from build123d import *

# Parameters (mm, degrees)
BOSS_EXTRUDE1_DEPTH = 15
CUT_EXTRUDE1_REACH  = 4
SKETCH3_R           = 1.5


with BuildPart() as part:
    # Sketch1 → Boss-Extrude1 (new body)
    with BuildSketch(Plane(origin=(0, 0, 0), x_dir=(0, 0, -1), z_dir=(1, 0, 0))):
        Polygon((0, 0), (16, 0), (16, -9), (26, -9), (26, -11), (14, -11), (14, -2), (0, -2), align=None)
    extrude(amount=-BOSS_EXTRUDE1_DEPTH)

    # Sketch3 → Cut-Extrude1 (cut, up to next)
    with BuildSketch(Plane(origin=(0, -9, 0), x_dir=(1, 0, 0), z_dir=(0, 1, 0)), mode=Mode.PRIVATE) as cut_extrude1_sk1:
        with Locations((-7.5, 21)):
            Circle(SKETCH3_R)
    cut_extrude1_tool1 = extrude(cut_extrude1_sk1.sketch, amount=-CUT_EXTRUDE1_REACH, mode=Mode.PRIVATE) & part.part
    add(cut_extrude1_tool1.solids().sort_by_distance((-7.5, -9, -21))[0], mode=Mode.SUBTRACT)


solid = part.part
The listing builds one solid part. Answer for the finished solid, in the listing's coordinates (mm). A direction names the side the tool comes from. Give positions to 0.01 mm unless a question says otherwise; leave off trailing zeros. Loops run counter-clockwise (first coordinate to the right, second up) from the corner with the lowest first, then second, coordinate; pieces in that order, holes last.
Item 1: A tool of negligible diameter and unlimited length cuts with its end or side. For faces 1 (the flat face through (-7, -2, -7)), 2 (the flat face through (-7, -4, -16)), 3 (the flat face through (-7, -10, -26)), from which of +Z, -Z, +X, -X, +Y, -Y can it reach the whole face along a straight path? Write none if from no direction.
Derived:
face 1: +Z, +X, -X, -Y
face 2: -Z, +X, -X, +Y
face 3: -Z, +X, -X, +Y, -Y
Item 2: Determine the mould class of faces 4 (the flat face through (-7, -1, 0)), 5 (the flat face through (-5.7, -9, -20.9)), 6 (the cylindrical face through (-8.61, -9.99, -22.01)) for opening direction Z: +Z half, -Z half, draft (parallel to the pull), parting line (faces both ways), or undercut.
Derived:
face 4: +Z half
face 5: draft
face 6: undercut
Item 3: A cutting plane is placed at A-A (x = -7.5). Give the vertices of the cut face in (y, z).
Derived:
outline: (-11, -26) - (-9, -26) - (-9, -22.5) - (-11, -22.5) - close; (-11, -19.5) - (-9, -19.5) - (-9, -16) - (0, -16) - (0, 0) - (-2, 0) - (-2, -14) - (-11, -14) - close
Item 4: A cutting plane is placed at C-C (x = -10). Give the vertices of the cut face in (y, z).
Derived:
outline: (-11, -26) - (-9, -26) - (-9, -16) - (0, -16) - (0, 0) - (-2, 0) - (-2, -14) - (-11, -14) - close
Item 5: A cutting plane is placed at D-D (y = -0.75). Give the vertices of the cut face in (x, z).
Derived:
outline: (-15, -16) - (0, -16) - (0, 0) - (-15, 0) - close
Item 6: Each of these flat-tipped pins is pushed along its axis until it touches: pin 1 Ø4 at (x, z) = (-4, -10) entering from -Y; pin 2 Ø8 at (x, z) = (-6, -21) entering from +Y; pin 3 Ø2 at (x, y) = (-7, -2.5) entering from +Z; pin 4 Ø2 at (x, y) = (-11, -5.5) entering from +Z. Where does it stop, or does it pass through?
Derived:
pin 1: stops at y = -2
pin 2: stops at y = -9
pin 3: stops at z = 0
pin 4: stops at z = -14
Item 7: A cutting plane is placed at B-B (z = -21). Give the vertices of the cut face in (x, y), then the cut area to 3 significant figures.
Derived:
outline: (-15, -11) - (-9, -11) - (-9, -9) - (-15, -9) - close; (-6, -11) - (0, -11) - (0, -9) - (-6, -9) - close
area: 24.0 mm2
Item 8: Find the intervals of material crossed by line 1 along X through (y, z) = (-9.7, -21); line 2 along Z through (x, y) = (-7.5, -9.5); line 3 along Y through (x, z) = (-12, -19.25), in increasing order.
Derived:
line 1: x = -15 to -9, -6 to 0
line 2: z = -26 to -22.5, -19.5 to -14
line 3: y = -11 to -9
